```python
from build123d import *

# Parameters (mm, degrees)
BOSS_EXTRUDE1_DEPTH = 14.5
SKETCH1_R           = 21.549999999999997
CUT_EXTRUDE1_DEPTH  = 1.95
BOSS_EXTRUDE3_START = 14.55
BOSS_EXTRUDE3_DEPTH = 16.5
SKETCH4_R           = 1.6999999999999995
CUT_EXTRUDE2_DEPTH  = 59.40978085903079
SKETCH5_R           = 3.2500000000000004
CUT_EXTRUDE3_DEPTH  = 4


with BuildPart() as part:
    # Sketch2 → Boss-Extrude1 (new body)
    with BuildSketch(Plane.XY):
        with BuildLine():
            Line((-20.50000000000001, -18.5), (-20.500000000000018, 34.34748899119118))
            ThreePointArc((-20.500000000000014, 34.347488991191184), (-19.7484176581315, -34.78505426185217), (40, -9.8e-15))
            ThreePointArc((40, 0), (34.785054261852174, 19.748417658131498), (20.500000000000004, 34.347488991191184))
            Line((20.5, 34.347488991191184), (20.5, -18.5))
            Line((20.500000000000004, -18.5), (-20.50000000000001, -18.5))
        make_face()
    extrude(amount=BOSS_EXTRUDE1_DEPTH)

    # Sketch1 → Cut-Extrude1 (cut)
    with BuildSketch(Plane.XY.offset(14.5)):
        Circle(SKETCH1_R)
    extrude(amount=-CUT_EXTRUDE1_DEPTH, mode=Mode.SUBTRACT)

    # Sketch1<3> → Boss-Extrude3 (add)
    with BuildSketch(Plane.XY.offset(14.5).offset(BOSS_EXTRUDE3_START)):
        with BuildLine():
            Line((20.5, -6.644734757685281), (20.5, -18.5))
            Line((20.5, -18.5), (11.052262211872641, -18.5))
            ThreePointArc((11.052262211872707, -18.500000000000284), (-5.0161e-13, -21.549999999999997), (-11.052262211873552, -18.49999999999978))
            Line((-11.0522622118736, -18.5), (-20.500000000000014, -18.5))
            Line((-20.50000000000001, -18.5), (-20.50000000000001, -6.644734757685747))
            ThreePointArc((-20.500000000000068, -6.644734757685756), (-21.549999999999997, 2.64e-15), (-20.500000000000064, 6.64473475768576))
            Line((-20.500000000000014, 6.644734757685754), (-20.500000000000018, 22.986735305389928))
            ThreePointArc((-20.499999999998952, 22.98673530538957), (-12.594443219135018, -28.107294426891826), (30.800000000000004, -7.54e-15))
            ThreePointArc((30.800000000000004, 0), (28.107294426892086, 12.594443219134437), (20.499999999999915, 22.98673530538871))
            Line((20.5, 22.98673530538874), (20.5, 6.644734757685303))
            ThreePointArc((20.500000000000203, 6.644734757685333), (21.285881471059685, 3.3635918301716967), (21.549999999999997, 0))
            ThreePointArc((21.549999999999997, -5.28e-15), (21.285881471059685, -3.3635918301717003), (20.500000000000206, -6.644734757685318))
        make_face()
        with BuildLine():
            Line((-20.500000000000014, -18.5), (-11.0522622118736, -18.5))
            ThreePointArc((-11.052262211873552, -18.49999999999978), (-16.852986120065246, -13.430538292893852), (-20.500000000000068, -6.644734757685756))
            Line((-20.50000000000001, -6.644734757685747), (-20.50000000000001, -18.5))
        make_face()
        with BuildLine():
            Line((11.052262211872641, -18.5), (20.5, -18.5))
            Line((20.5, -18.5), (20.5, -6.644734757685281))
            ThreePointArc((20.500000000000206, -6.644734757685318), (16.852986120065083, -13.430538292894052), (11.052262211872707, -18.500000000000284))
        make_face()
    extrude(amount=-BOSS_EXTRUDE3_DEPTH)

    # Sketch4 → Cut-Extrude2 (cut, through all)
    with BuildSketch(Plane.XY.offset(14.5)):
        with Locations((30, 18.508444018879594)):
            Circle(SKETCH4_R)
        with Locations((30, -18.508444018879594)):
            Circle(SKETCH4_R)
        with Locations((-30, 18.508444018879594)):
            Circle(SKETCH4_R)
        with Locations((-30, -18.508444018879594)):
            Circle(SKETCH4_R)
    extrude(amount=-CUT_EXTRUDE2_DEPTH, mode=Mode.SUBTRACT)

    # Sketch5 → Cut-Extrude3 (cut)
    with BuildSketch(Plane.XY.offset(14.5)):
        with Locations((-30, 18.508444018879594)):
            Circle(SKETCH5_R)
        with Locations((30, 18.508444018879594)):
            Circle(SKETCH5_R)
        with Locations((30, -18.508444018879594)):
            Circle(SKETCH5_R)
        with Locations((-30, -18.508444018879594)):
            Circle(SKETCH5_R)
    extrude(amount=-CUT_EXTRUDE3_DEPTH, mode=Mode.SUBTRACT)


solid = part.part
```
Verification items for the finished model (mm, model axes). A direction names the side the tool comes from. Coordinates: 2 decimals unless noted, no trailing zeros. Loops run counter-clockwise (first coordinate to the right, second up) from the corner with the lowest first, then second, coordinate; pieces in that order, holes last. Notation, with made-up numbers: (50, 84) - (65, 84) arc R9 cw to (65, 89) - close; hole circle Ø9 at (52.25, -36). An arc over 180 degrees is marked (long way). Answer as a JSON object with one key per item and string values.
(1) Cross-section at B-B, the plane x = 0. Record the boundary of the cut face in (y, z).
Response:
{"outline": "(-40, 0) - (-18.5, 0) - (-18.5, 12.55) - (-21.55, 12.55) - (-21.55, 29.05) - (-30.8, 29.05) - (-30.8, 14.5) - (-40, 14.5) - close"}
(2) Mould release check, pull along Y, two halves, no side actions. Record for faces 4 (the cylindrical face through (-1.458, -39.973, 7.148)), 5 (the flat face through (-5, -22, 29.05)), 6 (the flat face through (31.4, -19.9, 10.5)): pulls with the +Y half, pulls with the -Y half, needs draft (parallel to the pull), parting line crosses it, or undercut.
Response:
{"face 4": "parting line crosses it", "face 5": "needs draft", "face 6": "undercut"}
(3) Go/stop test with flat-tipped pins: pin 1 Ø7 at (x, y) = (-30, -17.5) entering from +Z; pin 2 Ø2 at (x, y) = (31, -18.5) entering from +Z; pin 3 Ø1 at (y, z) = (-1.5, 14.5) entering from +X; pin 4 Ø2 at (x, y) = (30, -18.51) entering from -Z. Record where each tip stops, or that it passes through.
Response:
{"pin 1": "stops at z = 14.5", "pin 2": "stops at z = 10.5", "pin 3": "stops at x = 39.99", "pin 4": "passes through"}
(4) Scan lines: line 1 along X through (y, z) = (-0.5, 23); line 2 along Y through (x, z) = (30, 13.25); line 3 along Y through (x, z) = (30, 4). Record each from-to range of solid material in increasing order.
Response:
{"line 1": "x = -30.8 to -21.54, 21.54 to 30.8", "line 2": "y = -26.46 to -21.76, -15.26 to 15.26, 21.76 to 26.46", "line 3": "y = -26.46 to -20.21, -16.81 to 16.81, 20.21 to 26.46"}
(5) Cross-section at C-C, the plane y = -1. Record the boundary of the cut face in (x, z), then the cut area to 3 significant figures.
Response:
{"outline": "(-39.99, 0) - (-20.5, 0) - (-20.5, 12.55) - (-21.53, 12.55) - (-21.53, 29.05) - (-30.78, 29.05) - (-30.78, 14.5) - (-39.99, 14.5) - close; (20.5, 0) - (39.99, 0) - (39.99, 14.5) - (30.78, 14.5) - (30.78, 29.05) - (21.53, 29.05) - (21.53, 12.55) - (20.5, 12.55) - close", "area": "831 mm²"}
(6) Cross-section at D-D, the plane z = 21.75. Record the boundary of the cut face in (x, y), then the cut area to 3 significant figures.
Response:
{"outline": "(-20.5, 6.64) - (-20.5, 22.99) arc R30.8 ccw (long way) to (20.5, 22.99) - (20.5, 6.64) arc R21.55 cw (long way) to start", "area": "1,080 mm²"}
(7) Cross-section at A-A, the plane y = 13.5. Record the boundary of the cut face in (x, z), then the cut area to 3 significant figures.
Response:
{"outline": "(-37.65, 0) - (-20.5, 0) - (-20.5, 29.05) - (-27.68, 29.05) - (-27.68, 14.5) - (-37.65, 14.5) - close; (20.5, 0) - (37.65, 0) - (37.65, 14.5) - (27.68, 14.5) - (27.68, 29.05) - (20.5, 29.05) - close", "area": "706 mm²"}
(8) Access from +Z, -Z, +X, -X, +Y, -Y to the whole of each face (thin tool, end or side, straight path). Record for faces 1 (the flat face through (-9, -30, 14.5)), 2 (the flat face through (0, -20, 12.55)), 3 (the flat face through (-18, -15, 12.55)).
Response:
{"face 1": "+Z", "face 2": "+Z, +Y", "face 3": "-Z, +Y"}
